from build123d import *

# Parameters (mm, degrees)
F0_W     = 609.6
F0_H     = 609.6
F1_DEPTH = 0.79375
F2_R     = 5.55625
F3_DEPTH = 25.4
F4_R     = 25.4
F4_R_2   = 4.7625
F5_DEPTH = 25.4


# Not quite as in the source:
# - a feature names something its author has since deleted; it is built from what else it names


with BuildPart() as f1:
    # F0 (on Front) → F1 (new body)
    with BuildSketch(Plane.XZ):
        with Locations((304.8, 304.8)):
            Rectangle(F0_W, F0_H)
    extrude(amount=F1_DEPTH)

    # F2 (on face) → F3 (cut)
    with BuildSketch(Plane.XZ.offset(0.79375)):
        with Locations((47.625, 355.6)):
            Circle(F2_R)
        with Locations((47.625, 152.4)):
            Circle(F2_R)
        with Locations((541.3375, 254)):
            Circle(F2_R)
        with Locations((541.3375, 457.2)):
            Circle(F2_R)
    extrude(amount=-F3_DEPTH, mode=Mode.SUBTRACT)

    # F4 (on face) → F5 (cut)
    with BuildSketch(Plane.XZ.offset(0.79375)):
        with Locations((495.3, 520.7)):
            Circle(F4_R)
        with Locations((508, 438.15)):
            Circle(F4_R_2)
        with Locations((508, 371.475)):
            Circle(F4_R_2)
    extrude(amount=-F5_DEPTH, mode=Mode.SUBTRACT)


solid = f1.part
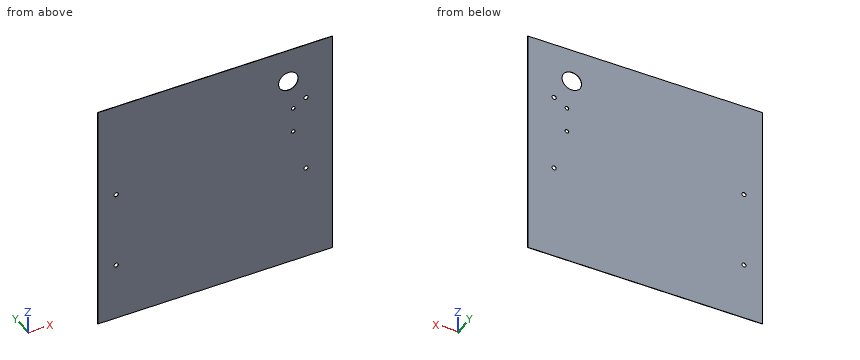
CAD build for the part. Positions are in the model's coordinates, mm. Coordinates: 2 decimals unless noted, no trailing zeros. Write each loop counter-clockwise with the first axis right and the second up, starting at its lowest first coordinate (ties: lowest second). Pieces come first, ordered by that corner, then holes. Notation, with made-up numbers: (72.25, -16.5) - (103.25, -16.5) arc R15 cw to (103.25, -12.5) - close; hole circle Ø11 at (63, 61). An arc over 180 degrees is marked (long way). Use a Markdown table: item, result. Add a question column.
Item 1: Drill centre lines: L1, parallel to X at y = -0.5, z = 152.5; L2, parallel to X at y = -0.3, z = 352; L3, parallel to Z at x = 515, y = -0.7. Where is each one in solid material? Low to high. Write a range as from..to.
Item 2: Band-saw the part on B-B, the plane x = 495.3. Give the cut face in (y, z).
Item 3: Band-saw the part on A-A, the plane z = 520.7. Give the cut face in (x, y), and give its area (3 significant figures).
Numbers:
| question | item | result |
|---|---|---|
| 1 | L1 | 0..42.07, 53.18..609.6 |
| 1 | L2 | 0..43.39, 51.86..609.6 |
| 1 | L3 | 0..504.67, 536.73..609.6 |
| 2 | outline | (-0.79, 0) - (0, 0) - (0, 495.3) - (-0.79, 495.3) - close; (-0.79, 546.1) - (0, 546.1) - (0, 609.6) - (-0.79, 609.6) - close |
| 3 | outline | (0, -0.79) - (469.9, -0.79) - (469.9, 0) - (0, 0) - close; (520.7, -0.79) - (609.6, -0.79) - (609.6, 0) - (520.7, 0) - close |
| 3 | area | 444 mm2 |
